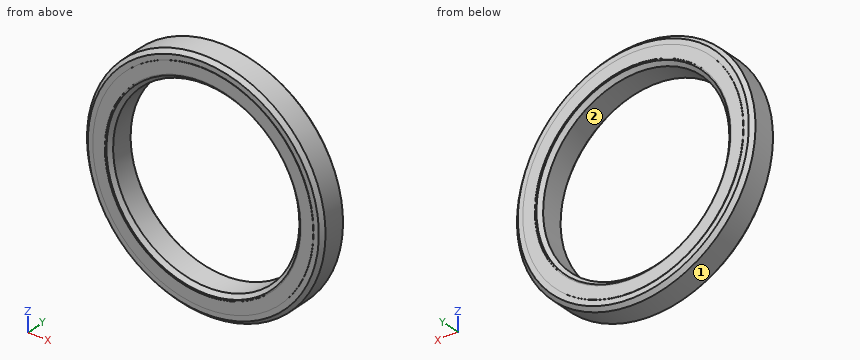
```python
from build123d import *

# Parameters (mm, degrees)
CROQUIS1_R              = 16
CROQUIS1_R_2            = 12.5
SALIENTE_EXTRUIR1_DEPTH = 2
CHAFL_N1_SIZE           = 0.5
CROQUIS2_R              = 14.793460403
CROQUIS2_R_2            = 13.169701353
SALIENTE_EXTRUIR2_DEPTH = 2.05


with BuildPart() as part:
    # Croquis1 → Saliente-Extruir1 (new, symmetric)
    with BuildSketch(Plane(origin=(0, 0, 0), x_dir=(1, 0, 0), z_dir=(0, 1, 0))):
        with Locations(Location((0, 0, 0), (0, 0, 270))):
            Circle(CROQUIS1_R)
        with Locations(Location((0, 0, 0), (0, 0, 270))):
            Circle(CROQUIS1_R_2, mode=Mode.SUBTRACT)
    extrude(amount=SALIENTE_EXTRUIR1_DEPTH, both=True)

    # Chaflán1
    chafl_n1_edges = [part.edges().sort_by_distance(p)[0] for p in [
        (0, -2, -16),
        (0, 2, -16),
        (0, -2, -12.5),
        (0, 2, -12.5),
    ]]
    chamfer(chafl_n1_edges, length=CHAFL_N1_SIZE)

    # Croquis2 → Saliente-Extruir2 (add, symmetric)
    with BuildSketch(Plane(origin=(0, 0, 0), x_dir=(1, 0, 0), z_dir=(0, 1, 0))):
        with Locations(Location((0, 0, 0), (0, 0, 270))):
            Circle(CROQUIS2_R)
        with Locations(Location((0, 0, 0), (0, 0, 270))):
            Circle(CROQUIS2_R_2, mode=Mode.SUBTRACT)
    extrude(amount=SALIENTE_EXTRUIR2_DEPTH, both=True)


solid = part.part
```
Work out the finished part from the listing and answer in its coordinate system (mm). Face numbers are marked on the shaded views. Give positions to 0.01 mm unless a question says otherwise; leave off trailing zeros. Write each loop counter-clockwise with the first axis right and the second up, starting at its lowest first coordinate (ties: lowest second). Pieces come first, ordered by that corner, then holes.
(1) The part is cut by section C-C on y = -0.45. Write down the section's boundary in (x, z).
Final values:
outline: circle Ø32 at (0, 0); hole circle Ø25 at (0, 0)
(2) Flat-ended cylindrical pins translate along their axes: pin 1 Ø1.5 at (x, y) = (8, -0.5) entering from +Z; pin 2 Ø1.5 at (y, z) = (1, 8) entering from +X; pin 3 Ø2 at (x, y) = (10, -1) entering from +Z. Find the tip coordinate at first contact, or state that the pin passes through.
Final values:
pin 1: stops at z = 14.26
pin 2: stops at x = 14.26
pin 3: stops at z = 13.23
(3) The mould has two halves that part along Z. Classify the marked faces 1 and 2: pulls with the +Z half, pulls with the -Z half, needs draft (parallel to the pull), parting line crosses it, or undercut.
Final values:
face 1: parting line crosses it
face 2: undercut
(4) Straight lines are drawn through the part: line 1 (X direction, y = -0.1, z = 0); line 2 (Z direction, x = 7.5, y = 1.95); line 3 (Z direction, x = 7, y = 1.85). For each, find the intervals that lie inside material, in ascending order.
Final values:
line 1: x = -16 to -12.5, 12.5 to 16
line 2: z = -13.62 to -10.56, 10.56 to 13.62
line 3: z = -14 to -10.78, 10.78 to 14
